from build123d import *

# Parameters (mm, degrees)
SKETCH_1_R      = 4
SKETCH_1_R_2    = 2.3
EXTRUDE_1_DEPTH = 1.25
FILLET_1_R      = 3


with BuildPart() as part:
    # 草图1 → 凸台-拉伸1 (new, symmetric)
    with BuildSketch(Plane.XY):
        with BuildLine():
            Line((-7, 4.82182538), (-7, 43))
            Line((-7, 43), (7, 43))
            Line((7, 43), (7, 4.82182538))
            ThreePointArc((7, 4.82182538), (0, -8.5), (-7, 4.82182538))
        make_face()
        Circle(SKETCH_1_R, mode=Mode.SUBTRACT)
        with Locations((0, 36)):
            Circle(SKETCH_1_R_2, mode=Mode.SUBTRACT)
        with Locations((0, 16)):
            Circle(SKETCH_1_R_2, mode=Mode.SUBTRACT)
    extrude(amount=EXTRUDE_1_DEPTH, both=True)

    # 圆角1
    fillet_1_edges = [part.edges().sort_by_distance(p)[0] for p in [
        (-7, 4.82182538, 0),
        (-7, 43, 0),
        (7, 43, 0),
        (7, 4.82182538, 0),
    ]]
    fillet(fillet_1_edges, radius=FILLET_1_R)


solid = part.part
For this review, take the finished solid that the model builds, in its own axes (mm). A direction names the side the tool comes from. Coordinates: 2 decimals unless noted, no trailing zeros. Order: outer loops, then holes, each group sorted by start corner. A loop starts at its lowest first (then second) coordinate and runs counter-clockwise, first axis right, second up. Notation, with made-up numbers: (6.25, 77.25) - (47.25, 77.25) arc R20 cw to (47.25, 106.25) - close; hole circle Ø3 at (82.25, -31). An arc over 180 degrees is marked (long way). Answer as CSV lines item,"result". Start each with the question number.
1) Add section C-C (z = -0.85). State the section outline as (x, y) points.
2) Machinability: for faces 1 (the flat face through (2, 18, -1.25)), 2 (the flat face through (-7, 23, 0)), which of the approach directions +Z, -Z, +X, -X, +Y, -Y give a long, thin tool a straight path to every point of the face, cutting with its end or side? Answer none if there is none.
3) Insertion check: P1, Ø1, axis at y = 27, z = -0.5, coming from the +X side; P2, Ø3, axis at x = 0, y = 16, coming from the +Z side; P3, Ø1.5, axis at y = 1.5, z = -1, coming from the -X side. Each pin has a flat end and moves straight along its axis. Give the tip position at first contact, or say it passes through.
4) To check wall thickness, follow line 1 along Y through (x, z) = (0, -0.7); line 2 along Y through (x, z) = (1.5, 0.8); line 3 along X through (y, z) = (30, 0.85). State the ranges of each line that lie inside material, in increasing order. Write a range as [from, to].
5) Add section D-D (y = 16.5). State the section outline as (x, z) points (3 decimals), then the cut area to 3 significant figures.
6) Add section A-A (y = 36). State the section outline as (x, z) points.
7) Add section B-B (x = 0). State the section outline as (y, z) points, then the cut area to 4 significant figures.
8) Draft analysis for pull direction Y (two halves, no side actions). For faces 3 (the cylindrical face through (-7.097, 4.923, 0.018)), 4 (the flat face through (7, 23, 0)), 5 (the cylindrical face through (0.248, -8.496, 0.018)), 6 (the cylindrical face through (-0.867, -3.905, -0.018)), state which applies: +Y half, -Y half, draft (parallel to the pull), parting line (faces both ways), or undercut.
Result:
1,outline,"(-7.39, 4.2) arc R8.5 ccw (long way) to (7.39, 4.2) arc R3 cw to (7, 5.68) - (7, 40) arc R3 ccw to (4, 43) - (-4, 43) arc R3 ccw to (-7, 40) - (-7, 5.68) arc R3 cw to start; hole circle Ø8 at (0, 0); hole circle Ø4.6 at (0, 16); hole circle Ø4.6 at (0, 36)"
2,face 1,"-Z, +X, -X, +Y, -Y"
2,face 2,"+Z, -Z, -X, +Y"
3,P1,"x = 7"
3,P2,"through"
3,P3,"x = -8.47"
4,line 1,"[-8.5, -4], [4, 13.7], [18.3, 33.7], [38.3, 43]"
4,line 2,"[-8.37, -3.71], [3.71, 14.26], [17.74, 34.26], [37.74, 43]"
4,line 3,"[-7, 7]"
5,outline,"(-7, -1.25) - (-2.245, -1.25) - (-2.245, 1.25) - (-7, 1.25) - close; (2.245, -1.25) - (7, -1.25) - (7, 1.25) - (2.245, 1.25) - close"
5,area,"23.8 mm^2"
6,outline,"(-7, -1.25) - (-2.3, -1.25) - (-2.3, 1.25) - (-7, 1.25) - close; (2.3, -1.25) - (7, -1.25) - (7, 1.25) - (2.3, 1.25) - close"
7,outline,"(-8.5, -1.25) - (-4, -1.25) - (-4, 1.25) - (-8.5, 1.25) - close; (4, -1.25) - (13.7, -1.25) - (13.7, 1.25) - (4, 1.25) - close; (18.3, -1.25) - (33.7, -1.25) - (33.7, 1.25) - (18.3, 1.25) - close; (38.3, -1.25) - (43, -1.25) - (43, 1.25) - (38.3, 1.25) - close"
7,area,"85.75 mm^2"
8,face 3,"+Y half"
8,face 4,"draft"
8,face 5,"parting line"
8,face 6,"undercut"
